Input: part model. Units: mm. Frame: model coordinates. A direction names the side the tool comes from. Round coordinates to 2 decimals unless told otherwise and drop trailing zeros. Loops run counter-clockwise (first coordinate to the right, second up) from the corner with the lowest first, then second, coordinate; pieces in that order, holes last. Notation, with made-up numbers: (44.25, 46) -> (48.25, 46) arc R26 cw to (48.25, 72) -> close; hole circle Ø6 at (3.5, -4.5). An arc over 180 degrees is marked (long way). One line per question, with ' | ' between items. Start each with the question number.
Q1. Material intervals for L1, parallel to X at y = 1.15, z = 0; L2, parallel to X at y = -4.25, z = -0.5; L3, parallel to Y at x = -13.5, z = -5.5, sorted ascending.
Q2. Cut plane A-A on z = 0. Return loops of the section in (x, y), and give its area (3 significant figures).
Q3. Cut plane D-D on x = -10. Return loops of the section in (y, z) (3 decimals), and give its area (3 significant figures).
Q4. Access query for faces 1 (the face through (15, 2.2, 0)), 2 (the face through (5, 6.7, 0)), 3 (the face through (-11.35, 4, 0)), 4 (the face through (15, 0, 0)), 5 (the face through (-15, 0, 0)). Directions: +Z, -Z, +X, -X, +Y, -Y. A direction counts if a zero-diameter tool reaches every point of the face in a straight line with its end or side. Return the directions, or none.
Q5. Cut plane B-B on x = -13.5. Return loops of the section in (y, z) (3 decimals).
Q6. Contact query for flat-ended pins moving along their axis: P1, Ø1.8, axis at x = -13.525, z = 0, coming from the -Y side; P2, Ø5, axis at y = -4.5, z = -3, coming from the +X side; P3, Ø4, axis at x = 4.5, z = -1, coming from the +Y side; P4, Ø4, axis at x = -14.5, z = 0.5, coming from the -Y side. Output: stop coordinate, or through.
Q7. Mould query, pull axis Z, two halves, no side actions, for faces 6 (the face through (-11.154, 8.736, -0.215)), 7 (the face through (11.35, 4, 0)), 8 (the face through (-12.55, 1.12, -0.04)). Classes: pulls with the +Z half, pulls with the -Z half, needs draft (parallel to the pull), parting line crosses it, or undercut.
Q8. Cut plane C-C on y = -11.25. Return loops of the section in (x, z) (3 decimals), and give its area (3 significant figures).
from build123d import *

# Parameters (mm, degrees)
SKETCH2_W                = 32.6
SKETCH2_H                = 11.85
BOSS_EXTRUDE2_DEPTH      = 2.2
SKETCH3_W                = 22.7
SKETCH3_H                = 11.85
BOSS_EXTRUDE3_DEPTH      = 4.5
BOSS_EXTRUDE3_DEPTH_BACK = 18.4
SKETCH4_R                = 0.975
CUT_EXTRUDE1_DEPTH       = 4.5
SKETCH5_R                = 5.75
SKETCH5_R_2              = 2.775
BOSS_EXTRUDE4_DEPTH      = 4.13


with BuildPart() as part:
    # Sketch2 → Boss-Extrude2 (new body)
    with BuildSketch(Plane(origin=(0, 0, 0), x_dir=(1, 0, 0), z_dir=(0, 1, 0))):
        Rectangle(SKETCH2_W, SKETCH2_H)
    extrude(amount=BOSS_EXTRUDE2_DEPTH)

    # Sketch3 → Boss-Extrude3 (add, two sides)
    with BuildSketch(Plane(origin=(0, 2.2, 0), x_dir=(1, 0, 0), z_dir=(0, 1, 0))) as boss_extrude3_sk:
        Rectangle(SKETCH3_W, SKETCH3_H)
    extrude(amount=BOSS_EXTRUDE3_DEPTH)
    extrude(boss_extrude3_sk.sketch, amount=-BOSS_EXTRUDE3_DEPTH_BACK)

    # Sketch4 → Cut-Extrude1 (cut)
    with BuildSketch(Plane(origin=(0, 2.2, 0), x_dir=(1, 0, 0), z_dir=(0, 1, 0))):
        with Locations((13.525, 0)):
            Circle(SKETCH4_R)
    cut_extrude1 = extrude(amount=-CUT_EXTRUDE1_DEPTH, mode=Mode.SUBTRACT)

    # Mirror1: Cut-Extrude1 across plane
    add(cut_extrude1.mirror(Plane(origin=(0, 0, 0), x_dir=(0, 0, 1), z_dir=(1, 0, 0))), mode=Mode.SUBTRACT)

    # Sketch5 → Boss-Extrude4 (add)
    with BuildSketch(Plane(origin=(0, 6.7, 0), x_dir=(1, 0, 0), z_dir=(0, 1, 0))):
        with Locations((-5.40813132, 0)):
            Circle(SKETCH5_R)
        with Locations((0.66686868, 0)):
            Circle(SKETCH5_R_2)
    extrude(amount=BOSS_EXTRUDE4_DEPTH)


solid = part.part
Results:
1) L1: -16.3 to -14.5, -12.55 to 12.55, 14.5 to 16.3 | L2: -11.35 to 11.35 | L3: 0 to 2.2
2) outline: (-16.3, 0) -> (-14.5, 0) -> (-14.5, 2.2) -> (-16.3, 2.2) -> close; (-12.55, 0) -> (-11.35, 0) -> (-11.35, -16.2) -> (11.35, -16.2) -> (11.35, 0) -> (12.55, 0) -> (12.55, 2.2) -> (11.35, 2.2) -> (11.35, 6.7) -> (3.44, 6.7) -> (3.44, 10.83) -> (-11.16, 10.83) -> (-11.16, 6.7) -> (-11.35, 6.7) -> (-11.35, 2.2) -> (-12.55, 2.2) -> close; (14.5, 0) -> (16.3, 0) -> (16.3, 2.2) -> (14.5, 2.2) -> close | area: 593 mm^2
3) outline: (-16.2, -5.925) -> (6.7, -5.925) -> (6.7, -3.461) -> (10.83, -3.461) -> (10.83, 3.461) -> (6.7, 3.461) -> (6.7, 5.925) -> (-16.2, 5.925) -> close | area: 300 mm^2
4) face 1: +Z, -Z, +X, +Y | face 2: +Y | face 3: +Z, -Z, -X, +Y | face 4: +Z, -Z, +X, -Y | face 5: +Z, -Z, -X, -Y
5) outline: (0, -5.925) -> (2.2, -5.925) -> (2.2, -0.975) -> (0, -0.975) -> close; (0, 0.975) -> (2.2, 0.975) -> (2.2, 5.925) -> (0, 5.925) -> close
6) P1: through | P2: x = 11.35 | P3: y = 10.83 | P4: y = 0
7) face 6: parting line crosses it | face 7: needs draft | face 8: undercut
8) outline: (-11.35, -5.925) -> (11.35, -5.925) -> (11.35, 5.925) -> (-11.35, 5.925) -> close | area: 269 mm^2
